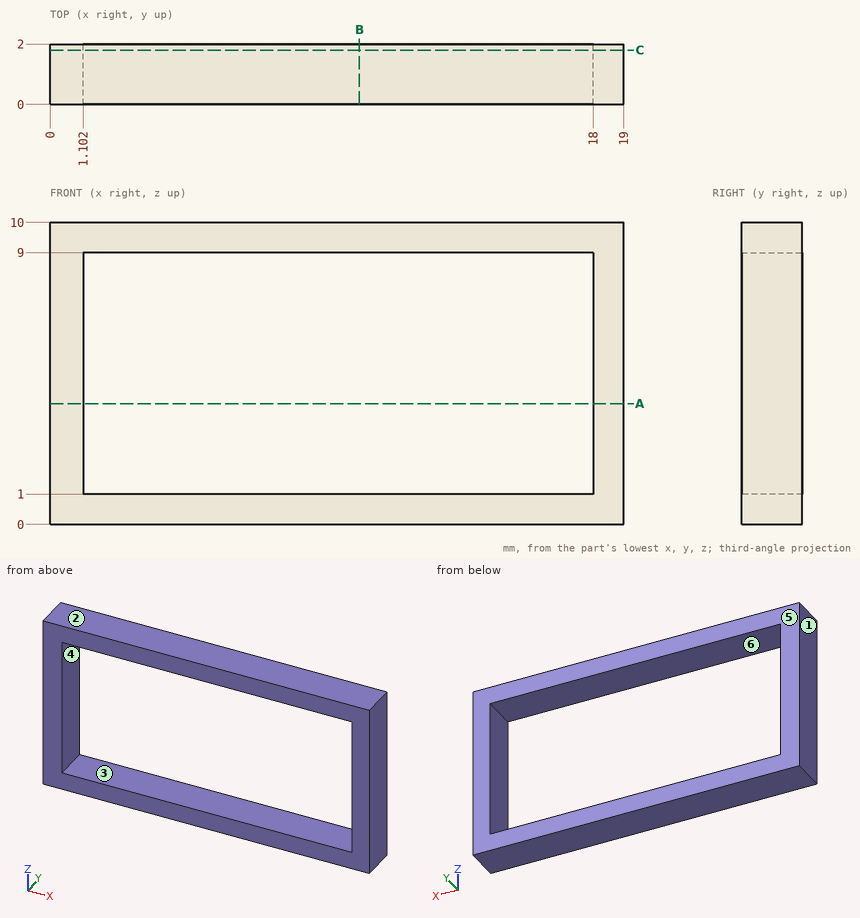
Answer from the drawing. Dimensions are ordinates in mm from the lowest x, y and z of the part. A direction names the side the tool comes from. Give positions to 0.01 mm unless a question says otherwise; leave off trailing zeros. Write each loop counter-clockwise with the first axis right and the second up, starting at its lowest first coordinate (ties: lowest second). Pieces come first, ordered by that corner, then holes.
1) Section A-A (z = 4) is taken. Write down the section's boundary in (x, y).
2) Find the intervals of material crossed by L1, parallel to X at y = 0.7, z = 8.25; L2, parallel to Z at x = 10.5, y = 0.6, in increasing order.
3) A tool of negligible diameter and unlimited length cuts with its end or side. For the marked faces 5 and 6, from which of +Z, -Z, +X, -X, +Y, -Y can it reach the whole face along a straight path? Write none if from no direction.
4) For a pull along X with two mould halves and no side action, classify the marked faces 1, 2, 3 and 4 as pulls with the +X half, pulls with the -X half, needs draft (parallel to the pull), parting line crosses it, or undercut.
5) Section B-B (x = 10.25) is taken. Write down the section's boundary in (y, z).
6) Given P1, Ø1, axis at y = 1.5, z = 4, coming from the -X side, flat-ended and moving along its own axis, determine where the tip first touches the part or whether it passes through.
7) Section C-C (y = 1.8) is taken. Write down the section's boundary in (x, z).
Response:
1. outline: (0, 0) - (1.1, 0) - (1.1, 2) - (0, 2) - close; (18, 0) - (19, 0) - (19, 2) - (18, 2) - close
2. L1: x = 0 to 1.1, 18 to 19
2. L2: z = 0 to 1, 9 to 10
3. face 5: +Z, -Z, +X, -X, +Y
3. face 6: +Y, -Y
4. face 1: pulls with the -X half
4. face 2: needs draft
4. face 3: undercut
4. face 4: undercut
5. outline: (0, 0) - (2, 0) - (2, 1) - (0, 1) - close; (0, 9) - (2, 9) - (2, 10) - (0, 10) - close
6. P1: stops at x = 0
7. outline: (0, 0) - (19, 0) - (19, 10) - (0, 10) - close; hole (1.1, 1) - (18, 1) - (18, 9) - (1.1, 9) - close
